```python
from build123d import *

# Parameters (mm, degrees)
SKETCH2_W           = 170
SKETCH2_H           = 35
BOSS_EXTRUDE1_DEPTH = 5
CUT_EXTRUDE1_DEPTH  = 200
SKETCH5_W           = 22
SKETCH5_H           = 5
BOSS_EXTRUDE2_DEPTH = 5
SKETCH6_W           = 22
SKETCH6_H           = 5
BOSS_EXTRUDE3_DEPTH = 5
CUT_EXTRUDE2_DEPTH  = 563


with BuildPart() as part:
    # Sketch2 → Boss-Extrude1 (new body)
    with BuildSketch(Plane(origin=(0, 0, 0), x_dir=(1, 0, 0), z_dir=(0, 1, 0))):
        Rectangle(SKETCH2_W, SKETCH2_H)
    extrude(amount=BOSS_EXTRUDE1_DEPTH)

    # Sketch4 → Cut-Extrude1 (cut)
    with BuildSketch(Plane.ZY.offset(85)):
        Polygon((-17.5, 0), (-12.5, 5), (-17.5, 5), align=None)
    extrude(amount=-CUT_EXTRUDE1_DEPTH, mode=Mode.SUBTRACT)

    # Sketch5 → Boss-Extrude2 (add)
    with BuildSketch(Plane.ZY.offset(85)):
        with Locations((2.5, 2.5)):
            Rectangle(SKETCH5_W, SKETCH5_H)
    extrude(amount=BOSS_EXTRUDE2_DEPTH)

    # Sketch6 → Boss-Extrude3 (add)
    with BuildSketch(Plane(origin=(85, 0, 0), x_dir=(0, 0, -1), z_dir=(1, 0, 0))):
        with Locations((-2.5, 2.5)):
            Rectangle(SKETCH6_W, SKETCH6_H)
    extrude(amount=BOSS_EXTRUDE3_DEPTH)

    # Sketch7 → Cut-Extrude2 (cut)
    with BuildSketch(Plane(origin=(85, 0, 0), x_dir=(0, 0, -1), z_dir=(1, 0, 0))):
        Polygon((12.5, 5), (10.5, 5), (15.5, 0), (17.5, 0), align=None)
    extrude(amount=-CUT_EXTRUDE2_DEPTH, mode=Mode.SUBTRACT)


solid = part.part
```
Work out the finished part from the listing and answer in its coordinate system (mm). A direction names the side the tool comes from. Round coordinates to 2 decimals unless told otherwise and drop trailing zeros. Loops run counter-clockwise (first coordinate to the right, second up) from the corner with the lowest first, then second, coordinate; pieces in that order, holes last. Notation, with made-up numbers: (83.25, 34.25) -> (123.25, 34.25) arc R23 ccw to (123.25, 69.25) -> close; hole circle Ø4 at (-34, 32). An arc over 180 degrees is marked (long way). Write each question's results on one line, items separated by ' | '. Start each with the question number.
1. Section A-A (y = 2.7) is taken. Determine the outline of the cut face in (x, z).
2. A tool of negligible diameter and unlimited length cuts with its end or side. For faces 1 (the face through (87, 2, -8.5)), 2 (the face through (-87, 2, 13.5)), 3 (the face through (87, 2, 13.5)), from which of +Z, -Z, +X, -X, +Y, -Y can it reach the whole face along a straight path? Write none if from no direction.
3. Section B-B (x = -48) is taken. Determine the outline of the cut face in (y, z), plus the area to 4 significant figures.
4. Given pin 1 Ø1.2 at (y, z) = (3.5, 15.5) entering from +X; pin 2 Ø3 at (y, z) = (2, 15.5) entering from -X; pin 3 Ø1.5 at (x, y) = (-88.5, 3.5) entering from -Z, each flat-ended and moving along its own axis, determine where each tip first touches the part or whether it passes through.
5. Find the intervals of material crossed by probe 1 along X at (y, z) = (3.85, 16.5); probe 2 along Z at (x, y) = (-66.5, 0.9); probe 3 along Z at (x, y) = (-8.5, 1.9), in increasing order. Write a range as from..to.
Evaluation:
1) outline: (-90, -8.5) -> (-85, -8.5) -> (-85, -12.8) -> (85, -12.8) -> (85, -8.5) -> (90, -8.5) -> (90, 13.5) -> (85, 13.5) -> (85, 17.5) -> (-85, 17.5) -> (-85, 13.5) -> (-90, 13.5) -> close
2) face 1: -Z, +X, +Y, -Y | face 2: +Z, -X, +Y, -Y | face 3: +Z, +X, +Y, -Y
3) outline: (0, -15.5) -> (5, -10.5) -> (5, 17.5) -> (0, 17.5) -> close | area: 152.5 mm2
4) pin 1: stops at x = 85 | pin 2: stops at x = -85 | pin 3: stops at z = -8.5
5) probe 1: x = -85..85 | probe 2: z = -14.6..17.5 | probe 3: z = -13.6..17.5
